```python
from build123d import *

# Parameters (mm, degrees)
SKETCH1_R           = 14.2875
BOSS_EXTRUDE1_DEPTH = 8
BOSS_EXTRUDE2_DEPTH = 44.45


with BuildPart() as part:
    # Sketch1 → Boss-Extrude1 (new body)
    with BuildSketch(Plane.XY):
        with BuildLine():
            Line((44.122092794, -38.1), (70.8, 0))
            Line((70.8, 0), (12.115221133, 26.66419084))
            ThreePointArc((12.115221133, 26.66419084), (6.19799028, 28.624160647), (0, 29.2875))
            Line((0, 29.2875), (-64.458376831, 29.2875))
            ThreePointArc((-64.458376831, 29.2875), (-70.622257624, -5.013654168), (-59.674366356, -38.1))
            Line((-59.674366356, -38.1), (44.122092794, -38.1))
        make_face()
        Circle(SKETCH1_R, mode=Mode.SUBTRACT)
    boss_extrude1 = extrude(amount=BOSS_EXTRUDE1_DEPTH)

    # Sketch1_3 → Boss-Extrude2 (add)
    with BuildSketch(Plane.XY):
        with BuildLine():
            Line((-59.674366356, -38.1), (-47.381747541, -38.1))
            ThreePointArc((-47.381747541, -38.1), (-58.074384746, -18.000162122), (-60.623939927, 4.62362495))
            ThreePointArc((-60.623939927, 4.62362495), (-58.272376031, 17.348492489), (-53.281163123, 29.2875))
            Line((-53.281163123, 29.2875), (-64.458376831, 29.2875))
            ThreePointArc((-64.458376831, 29.2875), (-69.196434445, 14.983105825), (-70.8, 0))
            ThreePointArc((-70.8, 0), (-67.96169928, -19.845589711), (-59.674366356, -38.1))
        make_face()
    extrude(amount=-BOSS_EXTRUDE2_DEPTH)

    # Mirror1: Boss-Extrude1 across plane
    add(boss_extrude1.mirror(Plane(origin=(0, 0, -22.225), x_dir=(1, 0, 0), z_dir=(0, 0, -1))))


solid = part.part
```
Source: CAD feature listing. Evaluate the final solid. Frame: model axes, mm. Give positions to 0.01 mm unless a question says otherwise; leave off trailing zeros. Loops run counter-clockwise (first coordinate to the right, second up) from the corner with the lowest first, then second, coordinate; pieces in that order, holes last. Notation, with made-up numbers: (4.25, 14) -> (38.25, 14) arc R18 cw to (38.25, 43) -> close; hole circle Ø11 at (87.5, 75.25). An arc over 180 degrees is marked (long way). Put each result on its own line as item: value. Start each with the question number.
1) Cut plane A-A (x = -36). Return loops of the section in (y, z), then the cut area to 3 significant figures.
2) Cut plane D-D (z = -40). Return loops of the section in (x, y), then the cut area to 3 significant figures.
3) Cut plane C-C (x = -1.5). Return loops of the section in (y, z).
4) Cut plane B-B (y = -12). Return loops of the section in (x, z).
5) Draft query along X for faces 1 (the face through (-54, 29.288, -24)), 2 (the face through (-14.274, 0.628, -48.394)), 3 (the face through (57.27, -19.32, -48.39)). Return one class per face: released by +X, released by -X, zero draft, split by the parting line, or undercut.
6) Material intervals for probe 1 along Y at (x, z) = (0, 3); probe 2 along Z at (x, y) = (36, -10.5); probe 3 along X at (y, z) = (-21, -29), sorted ascending.
Results are:
1. outline: (-38.1, -52.45) -> (29.29, -52.45) -> (29.29, -44.45) -> (-38.1, -44.45) -> close; (-38.1, 0) -> (29.29, 0) -> (29.29, 8) -> (-38.1, 8) -> close
1. area: 1,080 mm2
2. outline: (-64.46, 29.29) arc R70.8 ccw to (-59.67, -38.1) -> (-47.38, -38.1) arc R60.8 cw to (-53.28, 29.29) -> close
2. area: 710 mm2
3. outline: (-38.1, -52.45) -> (-14.21, -52.45) -> (-14.21, -44.45) -> (-38.1, -44.45) -> close; (-38.1, 0) -> (-14.21, 0) -> (-14.21, 8) -> (-38.1, 8) -> close; (14.21, -52.45) -> (29.29, -52.45) -> (29.29, -44.45) -> (14.21, -44.45) -> close; (14.21, 0) -> (29.29, 0) -> (29.29, 8) -> (14.21, 8) -> close
4. outline: (-69.78, -52.45) -> (-7.75, -52.45) -> (-7.75, -44.45) -> (-59.6, -44.45) -> (-59.6, 0) -> (-7.75, 0) -> (-7.75, 8) -> (-69.78, 8) -> close; (7.75, -52.45) -> (62.4, -52.45) -> (62.4, -44.45) -> (7.75, -44.45) -> close; (7.75, 0) -> (62.4, 0) -> (62.4, 8) -> (7.75, 8) -> close
5. face 1: zero draft
5. face 2: undercut
5. face 3: released by +X
6. probe 1: y = -38.1 to -14.29, 14.29 to 29.29
6. probe 2: z = -52.45 to -44.45, 0 to 8
6. probe 3: x = -67.61 to -57.06
